Part model, mm, in its own coordinate system. A direction names the side the tool comes from. Coordinates: 2 decimals unless noted, no trailing zeros. Write each loop counter-clockwise with the first axis right and the second up, starting at its lowest first coordinate (ties: lowest second). Pieces come first, ordered by that corner, then holes. Notation, with made-up numbers: M 1.5,83 L 39.5,83 A17 cw 39.5,89 Z; hole C -19,-10 d3. An arc over 180 degrees is marked long. Use a Markdown table: item, result. Add a question column.
Q1. Slice it at C-C on z = 35. Write the cut outline in (x, y).
Q2. Tool access for faces 1 (the flat face through (17, -21, 0)), 2 (the cylindrical face through (28.14, 8.86, 6.97)): list every direction of +Z, -Z, +X, -X, +Y, -Y with a clear straight run to the whole face (end or side of a thin tool).
Q3. Mould opens along X. For faces 3 (the cylindrical face through (25.467, 8.02, 5.226)), 4 (the flat face through (0, -30, 9)), 5 (the conical face through (-26.68, -20.46, 16.32)) say: released by +X, released by -X, zero draft, split by the parting line, or undercut.
Q4. Slice it at A-A on x = 0. Write the cut outline in (y, z), then the cut area to 3 significant figures.
Q5. Pin check, flat tips, straight feed: pin 1 Ø10 at (y, z) = (6.5, 14.5) entering from +X; pin 2 Ø2 at (y, z) = (31, 27.5) entering from +X; pin 3 Ø2 at (y, z) = (16.5, 24.5) entering from +X. Stop position of each tip, or through.
Q6. Wall check: L1, parallel to Y at x = 0, z = 6; L2, parallel to X at y = 33.5, z = 28.5; L3, parallel to X at y = -24.5, z = 30. Give the ranges that are in metal, low to high. Write a range as from..to.
from build123d import *


with BuildPart() as part:
    # Sketch → Revolution (revolve)
    with BuildSketch(Plane.XZ):
        with BuildLine():
            Line((28.3, 0), (28.3, 5))
            Line((29.5, 5), (28.3, 5))
            Line((29.5, 9), (29.5, 5))
            Line((29.5, 9), (33.7, 9))
            ThreePointArc((33.7, 9), (34.3, 9.6), (33.7, 10.2))
            ThreePointArc((31.847889, 12.677454), (32.556883, 11.276455), (33.7, 10.2))
            ThreePointArc((32.472114, 15.172114), (31.814653, 14.011199), (31.847889, 12.677454))
            Line((56.2, 38.9), (32.472114, 15.172114))
            Line((55, 38.9), (56.2, 38.9))
            Line((26.7, 10.6), (55, 38.9))
            Line((26.7, 10.6), (26.7, 0))
            Line((26.7, 0), (28.3, 0))
        make_face()
    revolve(axis=Axis((0, 0, 0), (0, 0, 1)))


solid = part.part
Recorded:
| question | item | result |
|---|---|---|
| 1 | outline | C 0,0 d104.6; hole C 0,0 d102.2 |
| 2 | face 1 | -Z, +X, -X, +Y, -Y |
| 2 | face 2 | -Z |
| 3 | face 3 | undercut |
| 3 | face 4 | zero draft |
| 3 | face 5 | split by the parting line |
| 4 | outline | M -56.2,38.9 L -32.47,15.17 A2.5 cw -31.85,12.68 A4.55 cw -33.7,10.2 A0.6 ccw -33.7,9 L -29.5,9 L -29.5,5 L -28.3,5 L -28.3,0 L -26.7,0 L -26.7,10.6 L -55,38.9 Z; M 26.7,0 L 28.3,0 L 28.3,5 L 29.5,5 L 29.5,9 L 33.7,9 A0.6 ccw 33.7,10.2 A4.55 cw 31.85,12.68 A2.5 cw 32.47,15.17 L 56.2,38.9 L 55,38.9 L 26.7,10.6 Z |
| 4 | area | 147 mm² |
| 5 | pin 1 | x = 36.29 |
| 5 | pin 2 | x = 33.99 |
| 5 | pin 3 | x = 39.57 |
| 6 | L1 | -29.5..-26.7, 26.7..29.5 |
| 6 | L2 | -31.23..-29.44, 29.44..31.23 |
| 6 | L3 | -40.46..-39.05, 39.05..40.46 |
